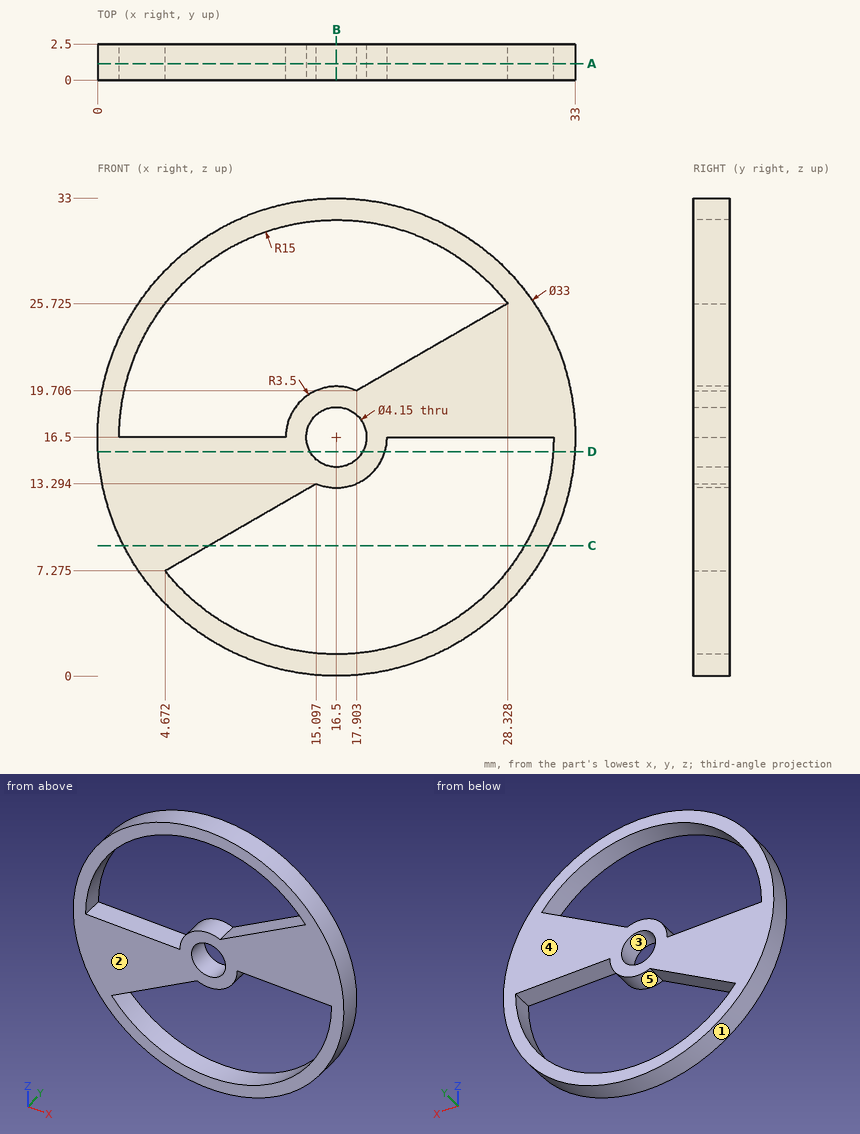
Check sheet for the drawn part. Datum: minimum x, y, z corner. Units: mm. A direction names the side the tool comes from. Round coordinates to 2 decimals unless told otherwise and drop trailing zeros. Order: outer loops, then holes, each group sorted by start corner. A loop starts at its lowest first (then second) coordinate and runs counter-clockwise, first axis right, second up. Notation, with made-up numbers: (83.25, -24.75) -> (136.25, -24.75) arc R15 ccw to (136.25, -5.75) -> close; hole circle Ø11 at (30.25, -26.5). An arc over 180 degrees is marked (long way). Return JSON: item names as keys, results as strings. Group by question number.
Q1. Tool access check on the marked faces 4 and 5. Record the directions out of +Z, -Z, +X, -X, +Y, -Y that give a thin tool (end or side, any length) a straight path to the whole face; none if there is none.
Q2. Section check A-A, the plane y = 1.15. Count the separate pieces of the cut face and the enclosed holes in it, plus the area to 3 significant figures.
Q3. Material ranges on probe 1 along X at (y, z) = (0.9, 15) (1 decimal); probe 2 along Z at (x, y) = (7, 0.8); probe 3 along X at (y, z) = (2.4, 17) (1 decimal), recorded low to high. Write a range as from..to.
Q4. Section check C-C, the plane z = 9. Record the boundary of the cut face in (x, y).
Q5. Release check for a two-part mould opening along X. For the marked faces 1, 2 and 3 record: released by +X, released by -X, zero draft, split by the parting line, or undercut.
Q6. Gauge pin test, flat ends, axial feed: pin 1 (1.2 mm diameter, centred on x = 5.5, y = 1.5, fed in from +Z); pin 2 (6 mm diameter, centred on x = 4, z = 18, fed in from +Y); pin 3 (1.2 mm diameter, centred on x = 25, y = 1, fed in from -Z) (1 decimal); pin 4 (3.5 mm diameter, centred on x = 16.5, z = 16.5, fed in from +Y). Record the tip position at first contact, or that the pin passes through.
Q7. Section check B-B, the plane x = 16.5. Record the boundary of the cut face in (y, z) (1 decimal).
Q8. Section check D-D, the plane z = 15.5. Record the boundary of the cut face in (x, y) (1 decimal).
Numbers:
{
 "1": {"face 4": "+Z, -Z, +X, -X, +Y", "face 5": "+Y, -Y"},
 "2": {"separate pieces": "1", "enclosed holes": "3", "area": "333 mm^2"},
 "3": {"probe 1": "0.1..15.1, 17.9..19.7, 31.4..32.9", "probe 2": "3.01..4.89, 8.62..16.5, 28.11..29.99", "probe 3": "0..1.5, 13..14.5, 18.5..33"},
 "4": {"outline": "(1.8, 0) -> (7.66, 0) -> (7.66, 2.5) -> (1.8, 2.5) -> close; (29.49, 0) -> (31.2, 0) -> (31.2, 2.5) -> (29.49, 2.5) -> close"},
 "5": {"face 1": "split by the parting line", "face 2": "zero draft", "face 3": "undercut"},
 "6": {"pin 1": "z = 29.31", "pin 2": "y = 2.5", "pin 3": "z = 2", "pin 4": "through"},
 "7": {"outline": "(0, 0) -> (2.5, 0) -> (2.5, 1.5) -> (0, 1.5) -> close; (0, 13) -> (2.5, 13) -> (2.5, 14.4) -> (0, 14.4) -> close; (0, 18.6) -> (2.5, 18.6) -> (2.5, 20) -> (0, 20) -> close; (0, 31.5) -> (2.5, 31.5) -> (2.5, 33) -> (0, 33) -> close"},
 "8": {"outline": "(0, 0) -> (14.7, 0) -> (14.7, 2.5) -> (0, 2.5) -> close; (18.3, 0) -> (19.9, 0) -> (19.9, 2.5) -> (18.3, 2.5) -> close; (31.5, 0) -> (33, 0) -> (33, 2.5) -> (31.5, 2.5) -> close"}
}
